Source: CAD feature listing. Evaluate the final solid. Frame: model axes, mm. A direction names the side the tool comes from. Round coordinates to 2 decimals unless told otherwise and drop trailing zeros. Order: outer loops, then holes, each group sorted by start corner. A loop starts at its lowest first (then second) coordinate and runs counter-clockwise, first axis right, second up. Notation, with made-up numbers: (-22.75, -29.5) -> (26.25, -29.5) arc R19 cw to (26.25, -7.5) -> close; hole circle Ø10 at (-12.75, -32). An arc over 180 degrees is marked (long way). One line per item, written item: value. Start each with the question number.
1) Ray query, L1, parallel to Y at x = 0, z = 8.25; L2, parallel to X at y = 0.25, z = 11.25; L3, parallel to X at y = -2.5, z = 9.5. Return the intervals inside material, ascending.
2) Section A-A (x = 0). Return the cut outline in (y, z).
3) Section C-C (z = 3.5). Return the cut outline in (x, y).
4) Mould query, pull axis X, two halves, no side actions, for faces 3 (the face through (11.923, 3.755, 5.916)), 4 (the face through (-8, 0, 10)), 5 (the face through (3, -3, 0)). Classes: pulls with the +X half, pulls with the -X half, needs draft (parallel to the pull), parting line crosses it, or undercut.
5) Reachability of faces 1 (the face through (3, -3, 12)), 2 (the face through (7.06, -0.91, 11.01)) from +Z, -Z, +X, -X, +Y, -Y: full face, straight path, thin tool, end or side. Return the list, or none.
6) Section D-D (x = 8.25). Return the cut outline in (y, z), and give its area (3 significant figures).
7) Pin query (flat end, axial travel): P1, Ø1.5, axis at x = 1, z = 10, coming from the +Y side; P2, Ø6, axis at y = -3.5, z = 11, coming from the -X side; P3, Ø3, axis at y = 4, z = 3.5, coming from the -X side. Return the tip coordinate at first contact, or that it passes through.
8) Section B-B (y = 0). Return the cut outline in (x, z), and give its area (3 significant figures).
```python
from build123d import *

# Parameters (mm, degrees)
ESQUISSE1_R             = 12.5
BOSS_EXTRU_1_DEPTH      = 12
ESQUISSE2_R             = 3
ENL_V_MAT_EXTRU_1_DEPTH = 12
ESQUISSE3_R             = 1.5
ENL_V_MAT_EXTRU_2_DEPTH = 2


with BuildPart() as part:
    # Esquisse1 → Boss.-Extru.1 (new body)
    with BuildSketch(Plane.XY):
        Circle(ESQUISSE1_R)
    extrude(amount=BOSS_EXTRU_1_DEPTH)

    # Esquisse2 → Enlèv. mat.-Extru.1 (cut)
    with BuildSketch(Plane.XY.offset(12)):
        Circle(ESQUISSE2_R)
    extrude(amount=-ENL_V_MAT_EXTRU_1_DEPTH, mode=Mode.SUBTRACT)

    # Esquisse3 → Enlèv. mat.-Extru.2 (cut)
    with BuildSketch(Plane.XY.offset(12)):
        with Locations((-8.25, 0)):
            Circle(ESQUISSE3_R)
        with Locations((8.25, 0)):
            Circle(ESQUISSE3_R)
    extrude(amount=-ENL_V_MAT_EXTRU_2_DEPTH, mode=Mode.SUBTRACT)


solid = part.part
```
Findings:
1. L1: -12.5 to -3, 3 to 12.5
1. L2: -12.5 to -9.73, -6.77 to -2.99, 2.99 to 6.77, 9.73 to 12.5
1. L3: -12.25 to -1.66, 1.66 to 12.25
2. outline: (-12.5, 0) -> (-3, 0) -> (-3, 12) -> (-12.5, 12) -> close; (3, 0) -> (12.5, 0) -> (12.5, 12) -> (3, 12) -> close
3. outline: circle Ø25 at (0, 0); hole circle Ø6 at (0, 0)
4. face 3: parting line crosses it
4. face 4: undercut
4. face 5: needs draft
5. face 1: +Z, +X, -X, +Y, -Y
5. face 2: +Z
6. outline: (-9.39, 0) -> (9.39, 0) -> (9.39, 12) -> (1.5, 12) -> (1.5, 10) -> (-1.5, 10) -> (-1.5, 12) -> (-9.39, 12) -> close
6. area: 219 mm2
7. P1: y = 12.5
7. P2: x = -12.49
7. P3: x = -12.25
8. outline: (-12.5, 0) -> (-3, 0) -> (-3, 12) -> (-6.75, 12) -> (-6.75, 10) -> (-9.75, 10) -> (-9.75, 12) -> (-12.5, 12) -> close; (3, 0) -> (12.5, 0) -> (12.5, 12) -> (9.75, 12) -> (9.75, 10) -> (6.75, 10) -> (6.75, 12) -> (3, 12) -> close
8. area: 216 mm2
